Could you check a few things on this model? Use its own coordinates, in mm. A direction names the side the tool comes from. Coordinates: 2 decimals unless noted, no trailing zeros. Order: outer loops, then holes, each group sorted by start corner. A loop starts at its lowest first (then second) coordinate and runs counter-clockwise, first axis right, second up. Notation, with made-up numbers: (31.25, 66) -> (86.25, 66) arc R33 ccw to (86.25, 97) -> close; hole circle Ø1 at (11, 61). An arc over 180 degrees is marked (long way). Use a Markdown table: item, result. Add a question column.
1) If we section it at A-A (x = 20): Write out the boundary of the cut face in (y, z), plus the area to 3 significant figures.
2) Will these pins go through, and if not, where does the flat tip stop? pin 1 Ø4 at (x, z) = (14, 14.5) entering from +Y; pin 2 Ø8 at (y, z) = (9.5, 3) entering from +X; pin 3 Ø5 at (x, y) = (-13.5, 14) entering from +Z; pin 4 Ø4 at (x, y) = (-15, 15) entering from +Z.
3) If we section it at C-C (y = 4): Write out the boundary of the cut face in (x, z).
4) Which directions (+Z, -Z, +X, -X, +Y, -Y) give clear straight access to the entire face, cutting with the end or side of a thin tool? Please do faces 4 (the cylindrical face through (0.37, 0.493, -19.997)), 5 (the cylindrical face through (0.66, 5.437, -14.985)).
5) If I drill on L1, parallel to Y at x = -1, z = 9.5; L2, parallel to Y at x = -21.5, z = -3; L3, parallel to X at y = 12.5, z = -7.5, over which ranges is the centre line in solid material (lowest first)? Write a range as [from, to].
6) Thinking about a two-plate mould opening in Z: for faces 1 (the cylindrical face through (-25, 0.5, -0.1)), 2 (the cylindrical face through (21.983, 0.493, -0.26)), 3 (the flat face through (0, 20, 0)), which applies, +Z half, -Z half, draft (parallel to the pull), parting line (faces both ways), or undercut?
7) If we section it at B-B (z = 0): Give the number of separate pieces and of enclosed holes in the cut face, plus the area to 3 significant figures.
8) If we section it at D-D (x = -21): Write out the boundary of the cut face in (y, z), plus the area to 3 significant figures.
```python
from build123d import *

# Parameters (mm, degrees)
SKETCH1_R           = 2
BOSS_EXTRUDE1_DEPTH = 1
SKETCH2_R           = 15
BOSS_EXTRUDE2_DEPTH = 14
FILLET1_R           = 5
SKETCH3_R           = 6
BOSS_EXTRUDE3_DEPTH = 5
FILLET2_R           = 5


with BuildPart() as part:
    # Sketch1 → Boss-Extrude1 (new body)
    with BuildSketch(Plane(origin=(0, 0, 0), x_dir=(1, 0, 0), z_dir=(0, 1, 0))):
        with BuildLine():
            ThreePointArc((-19.375, -4.960783708), (0, -20), (19.375, -4.960783708))
            ThreePointArc((19.375, -4.960783708), (25, 0), (19.375, 4.960783708))
            ThreePointArc((19.375, 4.960783708), (0, 20), (-19.375, 4.960783708))
            ThreePointArc((-19.375, 4.960783708), (-25, 0), (-19.375, -4.960783708))
        make_face()
        with Locations(Location((-20, 0, 0), (0, 0, 270))):
            Circle(SKETCH1_R, mode=Mode.SUBTRACT)
        with Locations(Location((20, 0, 0), (0, 0, 270))):
            Circle(SKETCH1_R, mode=Mode.SUBTRACT)
    extrude(amount=BOSS_EXTRUDE1_DEPTH)

    # Sketch2 → Boss-Extrude2 (add)
    with BuildSketch(Plane(origin=(0, 1, 0), x_dir=(1, 0, 0), z_dir=(0, 1, 0))):
        with Locations(Location((0, 0, 0), (0, 0, 270))):
            Circle(SKETCH2_R)
    extrude(amount=BOSS_EXTRUDE2_DEPTH)

    # Fillet1
    fillet1_edges = [part.edges().sort_by_distance(p)[0] for p in [
        (0, 15, -15),
    ]]
    fillet(fillet1_edges, radius=FILLET1_R)

    # Sketch3 → Boss-Extrude3 (add)
    with BuildSketch(Plane(origin=(0, 15, 0), x_dir=(1, 0, 0), z_dir=(0, 1, 0))):
        with Locations(Location((0, 0, 0), (0, 0, 270))):
            Circle(SKETCH3_R)
    extrude(amount=BOSS_EXTRUDE3_DEPTH)

    # Fillet2
    fillet2_edges = [part.edges().sort_by_distance(p)[0] for p in [
        (0, 20, -6),
    ]]
    fillet(fillet2_edges, radius=FILLET2_R - 0.0001)  # a hair under: the kernel refuses the full size


solid = part.part
```
Answer sheet:
| question | item | result |
|---|---|---|
| 1 | outline | (0, -5) -> (1, -5) -> (1, -2) -> (0, -2) -> close; (0, 2) -> (1, 2) -> (1, 5) -> (0, 5) -> close |
| 1 | area | 6.00 mm2 |
| 2 | pin 1 | y = 1 |
| 2 | pin 2 | x = 15 |
| 2 | pin 3 | z = 8.55 |
| 2 | pin 4 | through |
| 3 | outline | circle Ø30 at (0, 0) |
| 4 | face 4 | -Z, +Y, -Y |
| 4 | face 5 | +Y |
| 5 | L1 | [0, 15] |
| 5 | L2 | [0, 1] |
| 5 | L3 | [-12.21, 12.21] |
| 6 | face 1 | parting line |
| 6 | face 2 | undercut |
| 6 | face 3 | draft |
| 7 | separate pieces | 3 |
| 7 | enclosed holes | 0 |
| 7 | area | 501 mm2 |
| 8 | outline | (0, -4.9) -> (1, -4.9) -> (1, -1.73) -> (0, -1.73) -> close; (0, 1.73) -> (1, 1.73) -> (1, 4.9) -> (0, 4.9) -> close |
| 8 | area | 6.33 mm2 |
